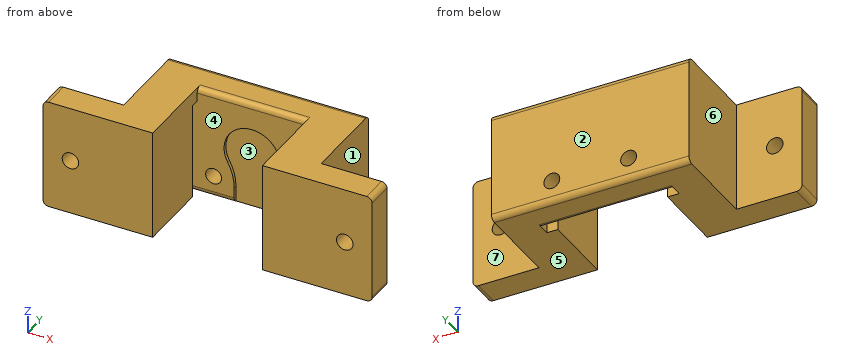
```python
from build123d import *

# Parameters (mm, degrees)
SKETCH1_W             = 20
SKETCH1_H             = 20
SKETCH1_R             = 1.5
BOSS_EXTRUDE1_DEPTH   = 5
BOSS_EXTRUDE1_2_DEPTH = 5
SKETCH2_W             = 8
SKETCH2_H             = 20
BOSS_EXTRUDE2_DEPTH   = 10
SKETCH3_W             = 20
SKETCH3_H             = 6
BOSS_EXTRUDE3_DEPTH   = 36
CUT_EXTRUDE1_DEPTH    = 0.6
SKETCH6_W             = 24.1
SKETCH6_H             = 1.6
CUT_EXTRUDE2_DEPTH    = 17.5
FILLET1_R             = 1
SKETCH8_R             = 1.45
CUT_EXTRUDE3_DEPTH    = 6
FILLET2_R             = 1


# Some blends are built 0.0001 mm under size
with BuildPart() as part:
    # Sketch1 → Boss-Extrude1 (new body)
    with BuildSketch(Plane(origin=(0, 0, 0), x_dir=(1, 0, 0), z_dir=(0, 1, 0))):
        with Locations((-17.614620188, -5)):
            Rectangle(SKETCH1_W, SKETCH1_H)
        with Locations(Location((-22.614620188, -5, 0), (0, 0, 270))):
            Circle(SKETCH1_R, mode=Mode.SUBTRACT)
    extrude(amount=BOSS_EXTRUDE1_DEPTH)



with BuildPart() as body_2:
    # Sketch1 → Boss-Extrude1 2 (new body)
    with BuildSketch(Plane(origin=(0, 0, 0), x_dir=(1, 0, 0), z_dir=(0, 1, 0))):
        with Locations((22.385379812, -5)):
            Rectangle(SKETCH1_W, SKETCH1_H)
        with Locations(Location((27.385379812, -5, 0), (0, 0, 270))):
            Circle(SKETCH1_R, mode=Mode.SUBTRACT)
    extrude(amount=BOSS_EXTRUDE1_2_DEPTH)


with BuildPart() as part_1:
    add(part.part)

    add(body_2.part)  # Boss-Extrude2 merges body 2
    # Sketch2 → Boss-Extrude2 (add)
    with BuildSketch(Plane(origin=(0, 5, 0), x_dir=(1, 0, 0), z_dir=(0, 1, 0))):
        with Locations((-11.614620188, -5)):
            Rectangle(SKETCH2_W, SKETCH2_H)
        with Locations((16.385379812, -5)):
            Rectangle(SKETCH2_W, SKETCH2_H)
    extrude(amount=BOSS_EXTRUDE2_DEPTH)

    # Sketch3 → Boss-Extrude3 (add)
    with BuildSketch(Plane.ZY.offset(15.614620188)):
        with Locations((5, 18)):
            Rectangle(SKETCH3_W, SKETCH3_H)
    extrude(amount=-BOSS_EXTRUDE3_DEPTH)

    # Sketch4 → Cut-Extrude1 (cut)
    with BuildSketch(Plane.XZ.offset(-15)):
        with BuildLine():
            Line((5.635379812, -2.069256579), (5.635379812, -13.54882393))
            Line((5.635379812, -13.54882393), (-0.864620188, -13.54882393))
            Line((-0.864620188, -13.54882393), (-0.864620188, -2.069256579))
            ThreePointArc((-0.864620188, -2.069256579), (-1.168628736, 0.293230663), (-2.06084614, 2.501785681))
            ThreePointArc((-2.06084614, 2.501785681), (2.385379812, 10.1), (6.831605764, 2.501785681))
            ThreePointArc((6.831605764, 2.501785681), (5.93938836, 0.293230663), (5.635379812, -2.069256579))
        make_face()
    extrude(amount=-CUT_EXTRUDE1_DEPTH, mode=Mode.SUBTRACT)

    # Sketch6 → Cut-Extrude2 (cut)
    with BuildSketch(Plane(origin=(0, 0, -5), x_dir=(-1, 0, 0), z_dir=(0, 0, -1))):
        with Locations((-2.335379812, 14.2)):
            Rectangle(SKETCH6_W, SKETCH6_H)
    extrude(amount=-CUT_EXTRUDE2_DEPTH, mode=Mode.SUBTRACT)

    # Fillet1
    fillet1_edges = [part_1.edges().sort_by_distance(p)[0] for p in [
        (2.385379812, 21, -5),
        (2.385379812, 21, 15),
        (32.385379812, 2.5, 15),
        (32.385379812, 2.5, -5),
        (-27.614620188, 2.5, -5),
        (-27.614620188, 2.5, 15),
    ]]
    fillet(fillet1_edges, radius=FILLET1_R)

    # Sketch8 → Cut-Extrude3 (cut)
    with BuildSketch(Plane(origin=(0, 15, 0), x_dir=(-1, 0, 0), z_dir=(0, -1, 0))):
        with Locations(Location((4.614620188, 1, 0), (0, 0, 90))):
            Circle(SKETCH8_R)
        with Locations(Location((-9.385379812, 1, 0), (0, 0, 90))):
            Circle(SKETCH8_R)
    extrude(amount=-CUT_EXTRUDE3_DEPTH, mode=Mode.SUBTRACT)

    # Fillet2
    fillet2_edges = [part_1.edges().sort_by_distance(p)[0] for p in [
        (2.385379812, 15, 15),
    ]]
    fillet(fillet2_edges, radius=FILLET2_R)
    # the kernel refuses this fillet: 1 mm, written as the material it takes off along each edge
    with BuildSketch(Plane(origin=(1.635379812, 15, -5), x_dir=(0, 0, 1), z_dir=(-1, 0, 0))) as fillet2_2_piece_1:
        with BuildLine():
            CenterArc((FILLET2_R, FILLET2_R), FILLET2_R, 180, 90)
            Line((0, FILLET2_R), (-FILLET2_R * 0.02, FILLET2_R))
            Line((-FILLET2_R * 0.02, FILLET2_R), (-FILLET2_R * 0.02, -FILLET2_R * 0.02))
            Line((-FILLET2_R * 0.02, -FILLET2_R * 0.02), (FILLET2_R, -FILLET2_R * 0.02))
            Line((FILLET2_R, -FILLET2_R * 0.02), (FILLET2_R, 0))
        make_face()
    extrude(amount=11.35, mode=Mode.SUBTRACT)
    fillet2_3_edges = [part_1.edges().sort_by_distance(p)[0] for p in [
        (10.010379812, 15, -5),
    ]]
    fillet(fillet2_3_edges, radius=FILLET2_R - 0.0001)  # a hair under: the kernel refuses the full size


solid = part_1.part
```
Work out the finished part from the listing and answer in its coordinate system (mm). Face numbers are marked on the shaded views. A direction names the side the tool comes from. Round coordinates to 2 decimals unless told otherwise and drop trailing zeros. Write each loop counter-clockwise with the first axis right and the second up, starting at its lowest first coordinate (ties: lowest second). Pieces come first, ordered by that corner, then holes. Notation, with made-up numbers: (25, 52) - (29, 52) arc R24 ccw to (29, 75) - close; hole circle Ø4 at (5.5, -29). An arc over 180 degrees is marked (long way). Return JSON: item names as keys, results as strings. Group by question number.
Q1. The part is cut by section D-D on y = 17.5. Write down the section's boundary in (x, z), then the cut area to 3 significant figures.
Q2. The part is cut by section C-C on z = 5. Write down the section's boundary in (x, y), then the cut area to 3 significant figures.
Q3. For the marked faces 5, 6 and 7, determine the directions among +Z, -Z, +X, -X, +Y, -Y from which every point of the face is accessible in a straight line to the end or side of a thin tool.
Q4. Each of these flat-tipped pins is pushed along its axis until it touches: pin 1 Ø4.5 at (x, z) = (-4.61, -1) entering from -Y; pin 2 Ø3 at (y, z) = (8.5, 7) entering from +X; pin 3 Ø5.5 at (x, z) = (0.5, 6) entering from -Y. Where does it stop, or does it pass through?
Q5. The part is cut by section A-A on y = 9.25. Write down the section's boundary in (x, z), then the cut area to 3 significant figures.
Q6. The mould has two halves that part along X. Classify the marked faces 1, 2, 3 and 4: released by +X, released by -X, zero draft, split by the parting line, or undercut.
Q7. The part is cut by section B-B on x = -8.5. Write down the section's boundary in (y, z), then the cut area to 3 significant figures.
Q8. Find the intervals of material crossed by L1, parallel to X at y = 18.7, z = -1; L2, parallel to X at y = 2.9, z = 5; L3, parallel to X at y = 11.5, z = 1, in increasing order.
Solved:
{
 "1": {"outline": "(-15.61, -5) - (20.39, -5) - (20.39, 15) - (-15.61, 15) - close; hole circle Ø2.9 at (-4.61, -1); hole circle Ø2.9 at (9.39, -1)", "area": "707 mm²"},
 "2": {"outline": "(-27.61, 0) - (-24.11, 0) - (-24.11, 5) - (-27.61, 5) - close; (-21.11, 0) - (-7.61, 0) - (-7.61, 13.4) - (-9.71, 13.4) - (-9.71, 15) - (-2.71, 15) - (-2.71, 15.6) - (7.49, 15.6) - (7.49, 15) - (14.39, 15) - (14.39, 13.4) - (12.39, 13.4) - (12.39, 0) - (25.89, 0) - (25.89, 5) - (20.39, 5) - (20.39, 21) - (-15.61, 21) - (-15.61, 5) - (-21.11, 5) - close; (28.89, 0) - (32.39, 0) - (32.39, 5) - (28.89, 5) - close", "area": "533 mm²"},
 "3": {"face 5": "-Z, +X, -X, +Y, -Y", "face 6": "+Z, -Z, -X, +Y", "face 7": "+Z, -Z, +X, +Y"},
 "4": {"pin 1": "y = 15", "pin 2": "x = 20.39", "pin 3": "y = 15.6"},
 "5": {"outline": "(-15.61, -5) - (-7.61, -5) - (-7.61, 15) - (-15.61, 15) - close; (12.39, -5) - (20.39, -5) - (20.39, 15) - (12.39, 15) - close", "area": "320 mm²"},
 "6": {"face 1": "released by +X", "face 2": "zero draft", "face 3": "undercut", "face 4": "undercut"},
 "7": {"outline": "(0, -5) - (13.4, -5) - (13.4, 12.5) - (15, 12.5) - (15, -4) arc R1 ccw to (16, -5) - (20, -5) arc R1 ccw to (21, -4) - (21, 14) arc R1 ccw to (20, 15) - (0, 15) - close", "area": "391 mm²"},
 "8": {"L1": "-15.61 to -6.06, -3.16 to 7.94, 10.84 to 20.39", "L2": "-27.61 to -24.11, -21.11 to -7.61, 12.39 to 25.89, 28.89 to 32.39", "L3": "-15.61 to -7.61, 12.39 to 20.39"}
}
